Autodesk Inventor part; units mm, degrees
ref_plane "YZ Plane" through (0, 0, 0) normal (1, 0, 0) x (0, 1, 0)
ref_plane "XZ Plane" through (0, 0, 0) normal (0, 1, 0) x (-1, 0, 0)
ref_plane "XY Plane" through (0, 0, 0) normal (0, 0, 1) x (1, 0, 0)
sketch "Skizze1" plane through (0, 0, 0) normal (0, 0, 1) x (1, 0, 0)
  line L0 (-20, 0) -> (120, 0)
  line L1 (0, -23) -> (0, 138)
  line L2 (0, 0) -> (100, 0)
  line L3 (100, 0) -> (100, 115)
  line L4 (100, 115) -> (0, 115)
  line L5 (0, 115) -> (0, 0)
  line L6 (5, 5) -> (95, 5)
  line L7 (95, 5) -> (95, 110)
  line L8 (95, 110) -> (5, 110)
  line L9 (5, 110) -> (5, 5)
  point P0 (0, 115)
  dimension "d0" = 5
  dimension "d1" = 5
  dimension "d2" = 5
  dimension "d3" = 5
  dimension "d4" = 90
  dimension "d5" = 105
extrude "Extrusion1" add sketch "Skizze1" along normal blind 100
sketch "Skizze2" plane through (0, 0, 100) normal (0, 0, 1) x (1, 0, 0)
  line L0 (0, 115) -> (0, 0)
  line L1 (0, 0) -> (100, 0)
  line L2 (100, 0) -> (100, 115)
  line L3 (100, 115) -> (0, 115)
  line L4 (0, 115) -> (0, 0)
extrude "Extrusion2" add sketch "Skizze2" along normal blind 5
sketch "Skizze3" plane through (0, 0, 105) normal (0, 0, 1) x (1, 0, 0)
  line L0 (100, 0) -> (100, 115)
  line L1 (100, 115) -> (0, 115)
  point P0 (0, 0)
  point P1 (50, 57.5)
  dimension "d10" = 50
  dimension "d11" = 57.5
hole "Bohrung1" at (50, 57.5, 105) direction (0, 0, -1) diameter 3 end through all
fillet "Rundung1" radius 0.4 1 edges at (50, 59, 105)
properties part number "Deckel_Koch_final" material "PMMA-Kunststoff"
Geometry check sheet. Reference: the model listing, model coordinates, mm. A direction names the side the tool comes from. Coordinates: 2 decimals unless noted, no trailing zeros. Order: outer loops, then holes, each group sorted by start corner. A loop starts at its lowest first (then second) coordinate and runs counter-clockwise, first axis right, second up. Notation, with made-up numbers: (71, 89) -> (87, 89) arc R28 ccw to (87, 121) -> close; hole circle Ø9 at (73, -25.5). An arc over 180 degrees is marked (long way). Use a Markdown table: item, result. Add a question column.
1. Cross-section at C-C (z = 19). Enter the section's corners in (x, y), and give its area (3 significant figures).
2. Go/stop test with flat-tipped pins: pin 1 Ø5 at (x, z) = (87, 13) entering from -Y; pin 2 Ø1.5 at (x, y) = (38.5, 62.5) entering from -Z. Record where each tip stops, or that it passes through.
3. Material ranges on L1, parallel to Y at x = 82.5, z = 27; L2, parallel to X at y = 57.5, z = 102.7; L3, parallel to Y at x = 50, z = 101.65, recorded low to high.
4. Cross-section at A-A (y = 57.5). Enter the section's corners in (x, z), and give its area (3 significant figures).
5. Mould release check, pull along Y, two halves, no side actions. Record for faces 3 (the face through (39, 58, 100)), 4 (the face through (49, 0, 52)), 5 (the face through (0, 57, 52)): pulls with the +Y half, pulls with the -Y half, needs draft (parallel to the pull), parting line crosses it, or undercut.
6. Set-up check for faces 1 (the face through (100, 57, 52)), 2 (the face through (49, 5, 49)): record each of +Z, -Z, +X, -X, +Y, -Y from which the full face is reachable in a straight line by a thin tool's end or side.
7. Cross-section at B-B (x = 50). Enter the section's corners in (y, z).
Filled sheet:
| question | item | result |
|---|---|---|
| 1 | outline | (0, 0) -> (100, 0) -> (100, 115) -> (0, 115) -> close; hole (5, 5) -> (95, 5) -> (95, 110) -> (5, 110) -> close |
| 1 | area | 2,050 mm2 |
| 2 | pin 1 | y = 0 |
| 2 | pin 2 | z = 100 |
| 3 | L1 | 0 to 5, 110 to 115 |
| 3 | L2 | 0 to 48.5, 51.5 to 100 |
| 3 | L3 | 0 to 56, 59 to 115 |
| 4 | outline | (0, 0) -> (5, 0) -> (5, 100) -> (48.5, 100) -> (48.5, 104.6) arc R0.4 ccw to (48.1, 105) -> (0, 105) -> close; (51.5, 100) -> (95, 100) -> (95, 0) -> (100, 0) -> (100, 105) -> (51.9, 105) arc R0.4 ccw to (51.5, 104.6) -> close |
| 4 | area | 1,480 mm2 |
| 5 | face 3 | undercut |
| 5 | face 4 | pulls with the -Y half |
| 5 | face 5 | needs draft |
| 6 | face 1 | +Z, -Z, +X, +Y, -Y |
| 6 | face 2 | -Z |
| 7 | outline | (0, 0) -> (5, 0) -> (5, 100) -> (56, 100) -> (56, 104.6) arc R0.4 ccw to (55.6, 105) -> (0, 105) -> close; (59, 100) -> (110, 100) -> (110, 0) -> (115, 0) -> (115, 105) -> (59.4, 105) arc R0.4 ccw to (59, 104.6) -> close |
